```python
from build123d import *

# Parameters (mm, degrees)
SKETCH1_W                              = 63.5
SKETCH1_H                              = 31.75
BOSS_EXTRUDE1_DEPTH                    = 120.65
HOLE1_D                                = 22.225
TAPPED_HOLE_FOR_10_32_HELICOIL3_REACH  = 120.859
TAPPED_HOLE_FOR_10_32_HELICOIL3_BORE_R = 2.5527
TAPPED_HOLE_FOR_10_32_HELICOIL4_D      = 5.1054
TAPPED_HOLE_FOR_10_32_HELICOIL5_D      = 5.1054
TAPPED_HOLE_FOR_10_32_HELICOIL5_DEPTH  = 17.018
TAPPED_HOLE_FOR_10_32_HELICOIL5_TIP    = 1.533816902


with BuildPart() as part:
    # Sketch1 → Boss-Extrude1 (new body)
    with BuildSketch(Plane(origin=(0, 0, 0), x_dir=(0, 0, -1), z_dir=(1, 0, 0))):
        Rectangle(SKETCH1_W, SKETCH1_H)
    extrude(amount=-BOSS_EXTRUDE1_DEPTH)

    # Hole1 (through all)
    with Locations(Plane.XY.offset(31.75)):
        with Locations((-60.325, -1.5875)):
            Hole(HOLE1_D / 2)

    # Tapped Hole for #10-32 Helicoil3 bore → Tapped Hole for #10-32 Helicoil3 (cut, up to next)
    with BuildSketch(Plane(origin=(-13.662401891, 15.875, 9.153963567), x_dir=(1, 0, 0), z_dir=(0, 1, 0)), mode=Mode.PRIVATE) as tapped_hole_for_10_32_helicoil3_sk1:
        with Locations((-46.662598109, 9.289125094)):
            Circle(TAPPED_HOLE_FOR_10_32_HELICOIL3_BORE_R)
    tapped_hole_for_10_32_helicoil3_tool1 = extrude(tapped_hole_for_10_32_helicoil3_sk1.sketch, amount=-TAPPED_HOLE_FOR_10_32_HELICOIL3_REACH, mode=Mode.PRIVATE) & part.part
    # Tapped Hole for #10-32 Helicoil3 bore → Tapped Hole for #10-32 Helicoil3 (cut, up to next)
    with BuildSketch(Plane(origin=(-13.662401891, 15.875, 9.153963567), x_dir=(1, 0, 0), z_dir=(0, 1, 0)), mode=Mode.PRIVATE) as tapped_hole_for_10_32_helicoil3_sk2:
        with Locations((-46.662598109, -9.760874906)):
            Circle(TAPPED_HOLE_FOR_10_32_HELICOIL3_BORE_R)
    tapped_hole_for_10_32_helicoil3_tool2 = extrude(tapped_hole_for_10_32_helicoil3_sk2.sketch, amount=-TAPPED_HOLE_FOR_10_32_HELICOIL3_REACH, mode=Mode.PRIVATE) & part.part
    add(tapped_hole_for_10_32_helicoil3_tool1.solids().sort_by_distance((-60.325, 15.875, -0.135162))[0], mode=Mode.SUBTRACT)
    add(tapped_hole_for_10_32_helicoil3_tool2.solids().sort_by_distance((-60.325, 15.875, 18.914838))[0], mode=Mode.SUBTRACT)

    # Tapped Hole for #10-32 Helicoil4 (through all)
    with Locations(Plane(origin=(0, 15.875, 0), x_dir=(1, 0, 0), z_dir=(0, 1, 0))):
        with Locations((-114.3, 15.875), (-114.3, -15.875), (-6.35, -15.875), (-6.35, 15.875)):
            Hole(TAPPED_HOLE_FOR_10_32_HELICOIL4_D / 2)

    # Tapped Hole for #10-32 Helicoil5
    with Locations(Plane(origin=(0, 15.875, 0), x_dir=(1, 0, 0), z_dir=(0, 1, 0))):
        with Locations((-80.9625, 22.225), (-39.6875, -22.225), (-80.9625, -22.225), (-39.6875, 22.225)):
            Hole(TAPPED_HOLE_FOR_10_32_HELICOIL5_D / 2, depth=TAPPED_HOLE_FOR_10_32_HELICOIL5_DEPTH)
            with Locations((0, 0, -(TAPPED_HOLE_FOR_10_32_HELICOIL5_DEPTH + TAPPED_HOLE_FOR_10_32_HELICOIL5_TIP / 2))):  # 118° drill point
                Cone(0, TAPPED_HOLE_FOR_10_32_HELICOIL5_D / 2, TAPPED_HOLE_FOR_10_32_HELICOIL5_TIP, mode=Mode.SUBTRACT)


solid = part.part
```
Here's how the part is built. I have some questions about the finished solid (model axes, mm). A direction names the side the tool comes from. Round coordinates to 2 decimals unless told otherwise and drop trailing zeros. Write each loop counter-clockwise with the first axis right and the second up, starting at its lowest first coordinate (ties: lowest second). Pieces come first, ordered by that corner, then holes.
Q1. Please list where these lines run through material, in increasing order: probe 1 along Z at (x, y) = (-114.3, 1.5); probe 2 along X at (y, z) = (-1.5, -14.5); probe 3 along X at (y, z) = (2, 24).
Q2. If we mould it in two halves opening along Z, with no side actions, what happens to faces 3 (the cylindrical face through (-42.122, 7.247, -22.992)), 4 (the flat face through (-59, 10, 31.75)), 5 (the flat face through (-120.65, 0, 0))? For each: +Z half, -Z half, draft (parallel to the pull), parting line (faces both ways), or undercut.
Q3. If we section it at D-D on x = -66: Write out the boundary of the cut face in (y, z) (3 decimals), plus the area to 3 significant figures.
Q4. Which directions (+Z, -Z, +X, -X, +Y, -Y) give clear straight access to the entire face, cutting with the end or side of a thin tool? Please do faces 1 (the cylindrical face through (-62.875, 12.598, -0.247)), 2 (the cylindrical face through (-112.42, -0.22, 14.15)).
Q5. If we section it at B-B on x = -6.35: Write out the boundary of the cut face in (y, z) (3 decimals).
Q6. Will these pins go through, and if not, where does the flat tip stop? P1, Ø4.5, axis at x = -114.3, z = 15.875, coming from the -Y side; P2, Ø4, axis at x = -60.32, z = 18.91, coming from the +Y side.
Q7. If we section it at C-C on y = -5.5: Write out the boundary of the cut face in (x, z) (3 decimals).
Q8. If we section it at A-A on y = 7: Give the number of separate pieces and of enclosed holes in the cut face, plus the area to 3 significant figures.
Answer below:
1. probe 1: z = -31.75 to -18.43, -13.32 to 13.32, 18.43 to 31.75
1. probe 2: x = -120.65 to -116.45, -112.15 to -71.44, -49.21 to -8.5, -4.2 to 0
1. probe 3: x = -120.65 to -82.8, -79.13 to -70.84, -49.81 to -41.52, -37.85 to 0
2. face 3: undercut
2. face 4: +Z half
2. face 5: draft
3. outline: (-15.875, -31.75) - (-11.142, -31.75) - (-11.142, 31.75) - (-15.875, 31.75) - close; (7.967, -31.75) - (15.875, -31.75) - (15.875, 31.75) - (7.967, 31.75) - close
3. area: 803 mm2
4. face 1: +Y
4. face 2: +Y, -Y
5. outline: (-15.875, -31.75) - (15.875, -31.75) - (15.875, -18.428) - (-15.875, -18.428) - close; (-15.875, -13.322) - (15.875, -13.322) - (15.875, 13.322) - (-15.875, 13.322) - close; (-15.875, 18.428) - (15.875, 18.428) - (15.875, 31.75) - (-15.875, 31.75) - close
6. P1: passes through
6. P2: stops at y = -12.52
7. outline: (-120.65, -31.75) - (-70.726, -31.75) - (-70.726, 31.75) - (-120.65, 31.75) - close; (-49.924, -31.75) - (0, -31.75) - (0, 31.75) - (-49.924, 31.75) - close; hole circle Ø5.105 at (-114.3, -15.875); hole circle Ø5.105 at (-114.3, 15.875); hole circle Ø5.105 at (-6.35, -15.875); hole circle Ø5.105 at (-6.35, 15.875)
8. separate pieces: 2
8. enclosed holes: 8
8. area: 6,600 mm2
